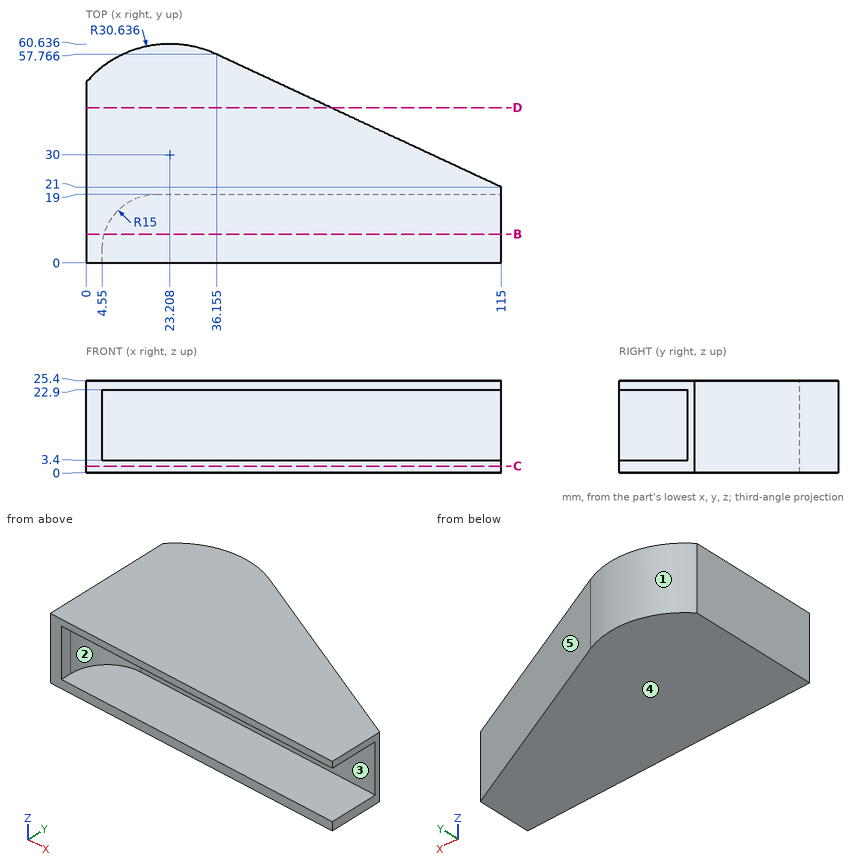
Design review of the part shown in the three views and the two pictorial views. Dimensions are in mm from the part's minimum x, y and z. A direction names the side the tool comes from. Round coordinates to 2 decimals unless told otherwise and drop trailing zeros. Order: outer loops, then holes, each group sorted by start corner. A loop starts at its lowest first (then second) coordinate and runs counter-clockwise, first axis right, second up. Notation, with made-up numbers: (32, -7) - (88, -7) arc R23 ccw to (88, 14) - close; hole circle Ø8 at (-24, 4.25). An arc over 180 degrees is marked (long way). One line per question, with ' | ' between items.
Item 1: Wall thickness on line 1 (Z direction, x = 32.5, y = 11); line 2 (Y direction, x = 43, z = 9.25) (1 decimal); line 3 (X direction, y = 52, z = 16.25) (1 decimal): over which ranges is each line inside the solid? List them lowest first. Write a range as [from, to].
Checks:
line 1: [0, 3.4], [22.9, 25.4] | line 2: [19, 54.6] | line 3: [1.9, 48.5]
Item 2: Machinability: for the marked faces 1 and 2, which of the approach directions +Z, -Z, +X, -X, +Y, -Y give a long, thin tool a straight path to every point of the face, cutting with its end or side? Answer none if there is none.
Checks:
face 1: +Z, -Z, +Y | face 2: +X, -Y
Item 3: Take a section at D-D, the plane y = 43. Write out the cut boundary in (x, z), then the cut area to 3 significant figures.
Checks:
outline: (0, 0) - (67.82, 0) - (67.82, 25.4) - (0, 25.4) - close | area: 1,720 mm²
Item 4: For P1, Ø10, axis at x = 60.5, z = 10, coming from the -Y side; P2, Ø1.2, axis at y = 1.5, z = 11.5, coming from the +X side; P3, Ø4, axis at y = 53.5, z = 17.5, coming from the -X side, all flat-tipped, find the tip position at first contact; note any pin that passes through.
Checks:
P1: y = 19 | P2: x = 4.55 | P3: x = 1.38
Item 5: Draft analysis for pull direction Z (two halves, no side actions). For the marked faces 3, 4 and 5, state which applies: +Z half, -Z half, draft (parallel to the pull), parting line (faces both ways), or undercut.
Checks:
face 3: undercut | face 4: -Z half | face 5: draft
Item 6: Take a section at B-B, the plane y = 8. Write out the cut boundary in (x, z).
Checks:
outline: (0, 0) - (115, 0) - (115, 3.4) - (5.09, 3.4) - (5.09, 22.9) - (115, 22.9) - (115, 25.4) - (0, 25.4) - close
Item 7: Take a section at C-C, the plane z = 1.75. Write out the cut boundary in (x, y) (1 decimal).
Checks:
outline: (0, 0) - (115, 0) - (115, 21) - (36.2, 57.8) arc R30.6 ccw to (0, 50) - close
